from build123d import *

# Parameters (mm, degrees)
BOSS_EXTRUDE1_DEPTH                     = 18
F_10_0MM_DOWEL_HOLE4_D                  = 9
CBORE_FOR_M5_HEX_HEAD_BOLT1_D           = 5
CBORE_FOR_M5_HEX_HEAD_BOLT1_CBORE_D     = 6
CBORE_FOR_M5_HEX_HEAD_BOLT1_CBORE_DEPTH = 13
CUT_EXTRUDE1_DEPTH                      = 20.0000001
CUT_EXTRUDE7_DEPTH                      = 10


with BuildPart() as part:
    # Sketch1 → Boss-Extrude1 (new body, symmetric)
    with BuildSketch(Plane.XY):
        with BuildLine():
            Line((22, 0), (22, 13))
            Line((22, 13), (50, 13))
            Line((50, 13), (50, 22))
            Line((50, 22), (25.690465157, 22))
            ThreePointArc((25.690465157, 22), (0, 32), (-25.690465157, 22))
            Line((-25.690465157, 22), (-50, 22))
            Line((-50, 22), (-50, 13))
            Line((-50, 13), (-22, 13))
            Line((-22, 13), (-22, 0))
            Line((-22, 0), (-18.027756377, 0))
            ThreePointArc((-18.027756377, 0), (0, 13), (18.027756377, 0))
            Line((18.027756377, 0), (22, 0))
        make_face()
    extrude(amount=BOSS_EXTRUDE1_DEPTH, both=True)

    # Ø10.0mm Dowel Hole4 (through all)
    with Locations(Plane(origin=(0, 22, 0), x_dir=(1, 0, 0), z_dir=(0, 1, 0))):
        with Locations((-31, 0)):
            f_10_0mm_dowel_hole4 = Hole(F_10_0MM_DOWEL_HOLE4_D / 2)

    # Mirror1: Ø10.0mm Dowel Hole4 across plane
    add(f_10_0mm_dowel_hole4.mirror(Plane(origin=(0, 0, 0), x_dir=(0, 0, 1), z_dir=(1, 0, 0))), mode=Mode.SUBTRACT)

    # CBORE for M5 Hex Head Bolt1 (through all)
    with Locations(Plane(origin=(0, 32, -0.198715446), x_dir=(1, 0, 0), z_dir=(0, 1, 0))):
        with Locations((0, 0)):
            CounterBoreHole(CBORE_FOR_M5_HEX_HEAD_BOLT1_D / 2, CBORE_FOR_M5_HEX_HEAD_BOLT1_CBORE_D / 2, CBORE_FOR_M5_HEX_HEAD_BOLT1_CBORE_DEPTH)

    # Sketch14 → Cut-Extrude1 (cut, through all)
    with BuildSketch(Plane.XZ.offset(-13)):
        with BuildLine():
            Line((-44.497190923, 18), (-50, 18))
            Line((-50, 18), (-50, -18))
            Line((-50, -18), (-44.359802254, -18.335974039))
            ThreePointArc((-44.359802254, -18.335974039), (-47.999656889, -0.181489808), (-44.497190923, 18))
        make_face()
        with BuildLine():
            Line((44.497190923, 18), (50, 18))
            Line((50, 18), (50, -18))
            Line((50, -18), (44.497190923, -18))
            ThreePointArc((44.497190923, -18), (48, 0), (44.497190923, 18))
        make_face()
    extrude(amount=-CUT_EXTRUDE1_DEPTH, mode=Mode.SUBTRACT)

    # Sketch17 → Cut-Extrude7 (cut)
    with BuildSketch(Plane(origin=(0, 22, 0), x_dir=(1, 0, 0), z_dir=(0, 1, 0))):
        with BuildLine():
            Line((-25.690465157, -6.637683312), (-25.690465157, 6.637683312))
            ThreePointArc((-25.690465157, 6.637683312), (-22.5, 0), (-25.690465157, -6.637683312))
        make_face()
    cut_extrude7 = extrude(amount=CUT_EXTRUDE7_DEPTH, mode=Mode.SUBTRACT)

    # Mirror3: Cut-Extrude7 across plane
    add(cut_extrude7.mirror(Plane(origin=(0, 0, 0), x_dir=(0, 0, 1), z_dir=(1, 0, 0))), mode=Mode.SUBTRACT)


solid = part.part
Design review of the part built by this model. Coordinates are the model's own, in mm. A direction names the side the tool comes from. Round coordinates to 2 decimals unless told otherwise and drop trailing zeros. Loops run counter-clockwise (first coordinate to the right, second up) from the corner with the lowest first, then second, coordinate; pieces in that order, holes last. Notation, with made-up numbers: M 53.25,-39 L 77.25,-39 A27 ccw 77.25,-13 Z; hole C 34,20.5 d7. An arc over 180 degrees is marked long. Answer as a JSON object with one key per item and string values.
Item 1: We need section C-C on y = 5. Give the boundary of the cut face in (x, z).
Answer sheet:
{"outline": "M -22,-18 L -15.49,-18 L -15.49,18 L -22,18 Z; M 15.49,-18 L 22,-18 L 22,18 L 15.49,18 Z"}
Item 2: Machinability: for faces 1 (the cylindrical face through (-22.5, 23, -0.1)), 2 (the flat face through (-22, 7, 0)), 3 (the cylindrical face through (22.5, 23, -0.1)), 4 (the cylindrical face through (-2.21, 25.59, -2.23)), 5 (the cylindrical face through (0.542, 15.872, 2.242)), which of the approach directions +Z, -Z, +X, -X, +Y, -Y give a long, thin tool a straight path to every point of the face, cutting with its end or side? Answer none if there is none.
Answer sheet:
{"face 1": "-X, +Y", "face 2": "+Z, -Z, -X, -Y", "face 3": "+X, +Y", "face 4": "+Y", "face 5": "+Y, -Y"}
Item 3: We need section B-B on z = 1. State how many separate pieces and enclosed holes the cut face has, and give its area (3 significant figures).
Answer sheet:
{"separate pieces": "4", "enclosed holes": "0", "area": "1,180 mm^2"}
Item 4: Clearance check with flat-ended pins moving along their axes: P1, Ø7.5, axis at x = -30.5, z = -7, coming from the +Y side; P2, Ø4, axis at x = -26, z = 11, coming from the -Y side; P3, Ø6, axis at x = 28.5, z = -14, coming from the +Y side. State where each tip first meets the part, or that it passes through.
Answer sheet:
{"P1": "stops at y = 22", "P2": "stops at y = 13", "P3": "stops at y = 22.17"}
Item 5: We need section D-D on y = 15.5. Give the boundary of the cut face in (x, z).
Answer sheet:
{"outline": "M -44.5,-18 L 44.5,-18 A48 ccw 44.5,18 L -44.5,18 A48 ccw Z; hole C -31,0 d9; hole C 0,-0.2 d5; hole C 31,0 d9"}
Item 6: Wall thickness on L1, parallel to Z at x = 31, y = 17.5; L2, parallel to X at y = 18.5, z = -2.5; L3, parallel to Z at x = 0, y = 15: over which ranges is each line inside the solid? List them lowest first. Write a range as from..to.
Answer sheet:
{"L1": "z = -18..-4.5, 4.5..18", "L2": "x = -47.93..-34.74, -27.26..-0.98, 0.98..27.26, 34.74..47.93", "L3": "z = -18..-2.7, 2.3..18"}
Item 7: The part is to be moulded in two halves that separate along Z. For faces 6 (the flat face through (22, 6, 0)), 7 (the cylindrical face through (-35.292, 17.437, -1.352)), 8 (the cylindrical face through (-48, 17, 0)), say which applies: pulls with the +Z half, pulls with the -Z half, needs draft (parallel to the pull), parting line crosses it, or undercut.
Answer sheet:
{"face 6": "needs draft", "face 7": "undercut", "face 8": "parting line crosses it"}
Item 8: We need section A-A on x = 0. Give the boundary of the cut face in (y, z), and give its area (3 significant figures).
Answer sheet:
{"outline": "M 13,-18 L 32,-18 L 32,-3.2 L 19,-3.2 L 19,-2.7 L 13,-2.7 Z; M 13,2.3 L 19,2.3 L 19,2.8 L 32,2.8 L 32,18 L 13,18 Z", "area": "576 mm^2"}
